Here's how the part is built. I have some questions about the finished solid (model axes, mm). A direction names the side the tool comes from. Coordinates: 2 decimals unless noted, no trailing zeros. Order: outer loops, then holes, each group sorted by start corner. A loop starts at its lowest first (then second) coordinate and runs counter-clockwise, first axis right, second up. Notation, with made-up numbers: (66.25, 21.5) - (98.25, 21.5) arc R28 ccw to (98.25, 49.5) - close; hole circle Ø5 at (52, 12.25). An arc over 180 degrees is marked (long way). Answer as CSV lines item,"result". Start each with the question number.
Q1. I need wall thicknesses on line 1 (X direction, y = 21, z = 38) (3 decimals); line 2 (Y direction, x = 38, z = 1); line 3 (Z direction, x = -32, y = -37) (3 decimals). Which ranges of each line are inside material? Lowest first, please.
Q2. Thinking about a two-plate mould opening in Y: for faces 1 (the face through (-1, 23, 0)), 2 (the face through (49.19, 1.377, 22.376)), which applies, released by +Y, released by -Y, zero draft, split by the parting line, or undercut?
Q3. For faces 3 (the face through (-1, 23, 3.175)), 4 (the face through (49, -4.762, 13)), 5 (the face through (34.93, 38.24, 1.61)), which set-ups out of +Z, -Z, +X, -X, +Y, -Y let a thin tool reach every point of the face, with its end or its side?
Q4. Suppose I cut it at B-B (x = -31.75). Please give me the cut outline in (y, z) (3 decimals).
Q5. Suppose I cut it at C-C (z = 42.5). Please give me the cut outline in (x, y) (1 decimal).
Q6. For pin 1 Ø10 at (x, y) = (-38.1, -38.1) entering from +Z (3 decimals); pin 2 Ø3.5 at (x, y) = (49, 14) entering from +Z; pin 3 Ø12 at (x, y) = (29.5, -33.5) entering from -Z; pin 4 Ø3.5 at (x, y) = (-48.5, -20.5) entering from +Z, each with a flat end and sliding along its axis, tell me the tip position at first contact or that it passes through.
Q7. Suppose I cut it at D-D (y = -31.75). Please give me the cut outline in (x, z) (3 decimals), then the cut area to 3 significant figures.
Q8. Suppose I cut it at A-A (x = 0). Please give me the cut outline in (y, z) (3 decimals), then the cut area to 3 significant figures.
from build123d import *

# Parameters (mm, degrees)
F0_W      = 101.6
F0_H      = 101.6
F1_DEPTH  = 3.175
F2_W      = 3.175
F2_H      = 101.6
F3_DEPTH  = 101.6
F4_W      = 3.175
F4_H      = 101.6
F5_DEPTH  = 101.6
F7_DEPTH  = 101.6
F8_R      = 6.35
F9_DEPTH  = 101.6
F11_DEPTH = 101.6
F12_R     = 3.175
F12_R_2   = 22.225
F13_DEPTH = 25.4


with BuildPart() as f1:
    # F0 (on Top) → F1 (new body)
    with BuildSketch(Plane.XY):
        Rectangle(F0_W, F0_H)
    extrude(amount=F1_DEPTH)

    # F2 (on face) → F3 (join)
    with BuildSketch(Plane.XY.offset(3.175)):
        with Locations((-49.2125, 0)):
            Rectangle(F2_W, F2_H)
    extrude(amount=F3_DEPTH)

    # F4 (on face) → F5 (join)
    with BuildSketch(Plane.XY.offset(3.175)):
        with Locations((49.2125, 0)):
            Rectangle(F4_W, F4_H)
    extrude(amount=F5_DEPTH)

    # F6 (on face) → F7 (cut)
    with BuildSketch(Plane(origin=(-50.8, 0, 0), x_dir=(0, -1, 0), z_dir=(-1, 0, 0))):
        with BuildLine():
            Line((-50.8, 104.775), (-50.8, 0))
            Line((-50.8, 0), (-11.779376, 96.822242))
            ThreePointArc((-11.779376, 96.822242), (-7.106336, 102.600682), (0, 104.775))
            Line((0, 104.775), (-50.8, 104.775))
        make_face()
        with BuildLine():
            Line((11.779376, 96.822242), (50.8, 0))
            Line((50.8, 0), (50.8, 104.775))
            Line((50.8, 104.775), (0, 104.775))
            ThreePointArc((0, 104.775), (7.106336, 102.600682), (11.779376, 96.822242))
        make_face()
    extrude(amount=-F7_DEPTH, mode=Mode.SUBTRACT)

    # F8 (on face) → F9 (cut)
    with BuildSketch(Plane(origin=(-50.8, 0, 0), x_dir=(0, -1, 0), z_dir=(-1, 0, 0))):
        with Locations((0, 28.575)):
            Circle(F8_R)
        with Locations((0, 92.075)):
            Circle(F8_R)
    extrude(amount=-F9_DEPTH, mode=Mode.SUBTRACT)

    # F10 (on face) → F11 (cut)
    with BuildSketch(Plane(origin=(-50.8, 0, 0), x_dir=(0, -1, 0), z_dir=(-1, 0, 0))):
        with BuildLine():
            ThreePointArc((4.7625, 40.348215), (6.59431, 39.428804), (8.25437, 38.226703))
            Line((8.25437, 38.226703), (22.205564, 45.470004))
            Line((22.205564, 45.470004), (7.541341, 81.856479))
            ThreePointArc((7.541341, 81.856479), (6.200838, 80.991697), (4.7625, 80.301785))
            Line((4.7625, 80.301785), (4.7625, 40.348215))
        make_face()
        with BuildLine():
            ThreePointArc((12.643355, 29.773157), (12.685831, 29.174748), (12.7, 28.575))
            ThreePointArc((12.7, 28.575), (12.685831, 27.975252), (12.643355, 27.376843))
            Line((12.643355, 27.376843), (33.957008, 16.311037))
            Line((33.957008, 16.311037), (25.782389, 36.594794))
            Line((25.782389, 36.594794), (12.643355, 29.773157))
        make_face()
        with BuildLine():
            ThreePointArc((-8.25437, 38.226703), (-6.59431, 39.428804), (-4.7625, 40.348215))
            Line((-4.7625, 40.348215), (-4.7625, 80.301785))
            ThreePointArc((-4.7625, 80.301785), (-6.200838, 80.991697), (-7.541341, 81.856479))
            Line((-7.541341, 81.856479), (-22.205564, 45.470004))
            Line((-22.205564, 45.470004), (-8.25437, 38.226703))
        make_face()
        with BuildLine():
            ThreePointArc((-12.643355, 27.376843), (-12.7, 28.575), (-12.643355, 29.773157))
            Line((-12.643355, 29.773157), (-25.782389, 36.594794))
            Line((-25.782389, 36.594794), (-33.957008, 16.311037))
            Line((-33.957008, 16.311037), (-12.643355, 27.376843))
        make_face()
        with BuildLine():
            Line((-4.7625, 9.525), (-4.7625, 16.801785))
            ThreePointArc((-4.7625, 16.801785), (-6.59431, 17.721196), (-8.25437, 18.923297))
            Line((-8.25437, 18.923297), (-26.356264, 9.525))
            Line((-26.356264, 9.525), (-4.7625, 9.525))
        make_face()
        with BuildLine():
            Line((26.356264, 9.525), (8.25437, 18.923297))
            ThreePointArc((8.25437, 18.923297), (6.59431, 17.721196), (4.7625, 16.801785))
            Line((4.7625, 16.801785), (4.7625, 9.525))
            Line((4.7625, 9.525), (26.356264, 9.525))
        make_face()
    extrude(amount=-F11_DEPTH, mode=Mode.SUBTRACT)

    # F12 (on face) → F13 (cut)
    with BuildSketch(Plane.XY.offset(3.175)):
        with Locations((38.1, 38.1)):
            Circle(F12_R)
        with Locations((31.75, 0)):
            Circle(F12_R)
        with Locations((38.1, -38.1)):
            Circle(F12_R)
        Circle(F12_R_2)
        with Locations((0, -31.75)):
            Circle(F12_R)
        with Locations((-31.75, 0)):
            Circle(F12_R)
        with Locations((0, 31.75)):
            Circle(F12_R)
        with Locations((-38.1, 38.1)):
            Circle(F12_R)
        with Locations((-38.1, -38.1)):
            Circle(F12_R)
    extrude(amount=-F13_DEPTH, mode=Mode.SUBTRACT)


solid = f1.part
Here are the results:
1,line 1,"x = -50.8 to -47.625, 47.625 to 50.8"
1,line 2,"y = -50.4 to -41.27, -34.93 to 34.93, 41.27 to 50.4"
1,line 3,"z = 0 to 3.175"
2,face 1,"zero draft"
2,face 2,"undercut"
3,face 3,"+Z, +Y, -Y"
3,face 4,"+X, -X"
3,face 5,"+Z, -Z"
4,outline,"(-50.8, 0) - (-3.175, 0) - (-3.175, 3.175) - (-49.52, 3.175) - close; (3.175, 0) - (50.8, 0) - (49.52, 3.175) - (3.175, 3.175) - close"
5,outline,"(-50.8, -33.7) - (-47.6, -33.7) - (-47.6, -16.5) - (-50.8, -16.5) - close; (-50.8, -4.8) - (-47.6, -4.8) - (-47.6, 4.8) - (-50.8, 4.8) - close; (-50.8, 16.5) - (-47.6, 16.5) - (-47.6, 33.7) - (-50.8, 33.7) - close; (47.6, -33.7) - (50.8, -33.7) - (50.8, -16.5) - (47.6, -16.5) - close; (47.6, -4.8) - (50.8, -4.8) - (50.8, 4.8) - (47.6, 4.8) - close; (47.6, 16.5) - (50.8, 16.5) - (50.8, 33.7) - (47.6, 33.7) - close"
6,pin 1,"stops at z = 3.175"
6,pin 2,"stops at z = 95.65"
6,pin 3,"stops at z = 0"
6,pin 4,"stops at z = 79.53"
7,outline,"(-50.8, 0) - (-3.175, 0) - (-3.175, 3.175) - (-47.625, 3.175) - (-47.625, 17.457) - (-50.8, 17.457) - close; (-50.8, 21.787) - (-47.625, 21.787) - (-47.625, 47.269) - (-50.8, 47.269) - close; (3.175, 0) - (50.8, 0) - (50.8, 17.457) - (47.625, 17.457) - (47.625, 3.175) - (3.175, 3.175) - close; (47.625, 21.787) - (50.8, 21.787) - (50.8, 47.269) - (47.625, 47.269) - close"
7,area,"555 mm²"
8,outline,"(-50.8, 0) - (-34.925, 0) - (-34.925, 3.175) - (-49.52, 3.175) - close; (-28.575, 0) - (-22.225, 0) - (-22.225, 3.175) - (-28.575, 3.175) - close; (22.225, 0) - (28.575, 0) - (28.575, 3.175) - (22.225, 3.175) - close; (34.925, 0) - (50.8, 0) - (49.52, 3.175) - (34.925, 3.175) - close"
8,area,"137 mm²"
